```python
from build123d import *

# Parameters (mm, degrees)
F1_DEPTH = 44.45
F2_T     = -3.175
F3_W     = 38.1
F3_H     = 38.3965011568
F4_DEPTH = 8.689331367
F6_D     = 6.7945


with BuildPart() as f1:
    # F0 (on Front) → F1 (new body)
    with BuildSketch(Plane.XZ):
        Polygon((-5.5562371184, -44.45), (17.9743102048, -44.45), (1223.1325170816, -44.45), (1228.6887542, 0), (0, 0), align=None)
    extrude(amount=F1_DEPTH)

    # F2
    f2_openings = [f1.faces().sort_by_distance(p)[0] for p in [
        (1225.910636, -22.225, -22.225),
    ]]
    offset(amount=F2_T, openings=f2_openings)

    # F3 (on face) → F4 (cut, through all)
    with BuildSketch(Plane(origin=(3.1504823709, 0, -0.3938093834), x_dir=(0, 1, 0), z_dir=(0.9922779121, 0, -0.1240344515))):
        with Locations((-22.225, -22.0010849282)):
            Rectangle(F3_W, F3_H)
    extrude(amount=-F4_DEPTH, mode=Mode.SUBTRACT)

    # F6 (through all)
    with Locations(Plane.XZ.offset(44.45)):
        with Locations((1092.1637542, -22.225)):
            Hole(F6_D / 2)


solid = f1.part
```
Input: part model. Units: mm. Frame: model coordinates. A direction names the side the tool comes from. Give positions to 0.01 mm unless a question says otherwise; leave off trailing zeros. Order: outer loops, then holes, each group sorted by start corner. A loop starts at its lowest first (then second) coordinate and runs counter-clockwise, first axis right, second up. Notation, with made-up numbers: (-17.5, 65) -> (9.5, 65) arc R26 cw to (9.5, 94) -> close; hole circle Ø3 at (57.25, 48.5). An arc over 180 degrees is marked (long way). Write each question's results on one line, items separated by ' | '. Start each with the question number.
Item 1: Cut plane A-A on x = 406. Return the cut outline in (y, z) (3 decimals), then the cut area to 3 significant figures.
Item 2: Mould query, pull axis Z, two halves, no side actions, for faces 3 (the flat face through (600, -22, -44.45)), 4 (the flat face through (-2.74, -2.16, -21.91)), 5 (the flat face through (602, -22, -41.275)). Classes: pulls with the +Z half, pulls with the -Z half, needs draft (parallel to the pull), parting line crosses it, or undercut.
Item 3: Line query: line 1 (Y direction, x = 1014, z = -34) (3 decimals). Output: solid intervals per line, ascending.
Item 4: Contact query for flat-ended pins moving along their axis: P1, Ø12, axis at y = -15.5, z = -38, coming from the +X side; P2, Ø6, axis at x = 1092.16, z = -22.22, coming from the +Y side. Output: stop coordinate, or through.
Item 5: Cut plane B-B on y = -29.5. Return the cut outline in (x, z) (3 decimals), then the cut area to 3 significant figures.
Item 6: Set-up query: faces 1 (the flat face through (1225.87, -2.16, -22.54)), 2 (the flat face through (624, -22, -3.175)). Return all of +Z, -Z, +X, -X, +Y, -Y with unobstructed straight access to the full face (end or side cutting, diameter ignored); none if empty.
Established:
1) outline: (-44.45, -44.45) -> (0, -44.45) -> (0, 0) -> (-44.45, 0) -> close; hole (-41.275, -41.275) -> (-3.175, -41.275) -> (-3.175, -3.175) -> (-41.275, -3.175) -> close | area: 524 mm^2
2) face 3: pulls with the -Z half | face 4: pulls with the +Z half | face 5: undercut
3) line 1: -44.45 to -41.275, -3.175 to 0
4) P1: x = 1223.53 | P2: through
5) outline: (-5.556, -44.45) -> (1223.133, -44.45) -> (1223.529, -41.275) -> (-1.96, -41.275) -> (-5.11, -40.881) -> close; (-0.348, -2.781) -> (2.803, -3.175) -> (1228.292, -3.175) -> (1228.689, 0) -> (0, 0) -> close | area: 7,800 mm^2
6) face 1: -Z, +X, +Y, -Y | face 2: +X, -X
